Can you work these out from the model? Positions are in its coordinate system, mm. A direction names the side the tool comes from. Coordinates: 2 decimals unless noted, no trailing zeros. Order: outer loops, then holes, each group sorted by start corner. A loop starts at its lowest first (then second) coordinate and runs counter-clockwise, first axis right, second up. Notation, with made-up numbers: (-27, 52.5) - (-9, 52.5) arc R9 ccw to (-9, 69.5) - close; hole circle Ø8 at (48, -9). An arc over 180 degrees is marked (long way). Return JSON: item names as keys, results as strings. Group by question number.
1) Imagine slicing it at D-D (y = 6). Write out the boundary of the cut face in (x, z).
2) If we mould it in two halves opening along Z, with no side actions, what happens to faces 4 (the face through (0, 5, 0)), 5 (the face through (1.74, 5.26, -2.52)), 6 (the face through (1.7, -3.1, 0.1))? For each: pulls with the +Z half, pulls with the -Z half, needs draft (parallel to the pull), parting line crosses it, or undercut.
3) If I drill on line 1 along Y through (x, z) = (1.5, 0); line 2 along Z through (x, y) = (1.4, 4.25); line 3 along X through (y, z) = (6, -0.5), over which ranges is the centre line in solid material (lowest first)?
4) Imagine slicing it at B-B (x = 0.5). Write out the boundary of the cut face in (y, z), and give its area (3 significant figures).
5) Imagine slicing it at A-A (x = 1.15). Write out the boundary of the cut face in (y, z).
6) For pin 1 Ø5 at (y, z) = (4.5, 1) entering from +X; pin 2 Ø3 at (y, z) = (-1.5, -3) entering from -X; pin 3 Ø2 at (x, z) = (1.5, 3) entering from -Y; pin 4 Ø0.8 at (x, y) = (1, -5) entering from -Z, each with a flat end and sliding along its axis, tell me the tip position at first contact or that it passes through.
7) Which directions (+Z, -Z, +X, -X, +Y, -Y) give clear straight access to the entire face, cutting with the end or side of a thin tool? Please do faces 1 (the face through (2, -5, 0)), 2 (the face through (1, -5, 1)), 3 (the face through (2, 5, 0)).
8) Imagine slicing it at C-C (z = -3.5). Write out the boundary of the cut face in (x, y), and give its area (3 significant figures).
```python
from build123d import *

# Parameters (mm, degrees)
CHAMFER_1_SIZE           = 0.5
CHAMFER_1_SIZE2          = 0.288675135
CUT_EXTRUDE_1_DEPTH      = 2.5
M3X0_51_AT_2_COUNT       = 2
M3X0_51_AT_2_PITCH       = 10
M3X0_51_AT_3_COUNT       = 2
M3X0_51_AT_3_PITCH       = 14.142135624
M3X0_51_AT_4_COUNT       = 2
M3X0_51_AT_4_PITCH       = 10
SKETCH_7_W               = 2
SKETCH_7_H               = 3
SKETCH_8_OUTSIDE_W       = 20.06
SKETCH_8_OUTSIDE_H       = 20.06
CUT_EXTRUDE_2_DEPTH      = 2.2
SKETCH_9_W               = 1.5
SKETCH_9_H               = 6
CUT_EXTRUDE_3_DEPTH      = 10
CUT_EXTRUDE_4_DEPTH      = 8
CUT_EXTRUDE_4_DEPTH_BACK = 8


with BuildPart() as part:
    # Эскиз1 → Повернуть1 (revolve)
    with BuildSketch(Plane.XY):
        Polygon((0, 1.5), (0, 10), (2, 10), (2, 4.5), (4.5, 4.5), (4.5, 2.5), (2, 2.5), (2, 3.1), (1, 3.1), (1, 1.5), align=None)
    revolve(axis=Axis((0, 0, 0), (1, 0, 0)))

    # Фаска1
    chamfer_1_edges = [part.edges().sort_by_distance(p)[0] for p in [
        (4.5, -2.5, 0),
    ]]
    chamfer_1_side = [part.faces().sort_by_distance(p)[0] for p in [
        (4.5, -4.372720779, 0),
    ]]
    chamfer(chamfer_1_edges, length=CHAMFER_1_SIZE, length2=CHAMFER_1_SIZE2, reference=chamfer_1_side[0])

    # Эскиз3 → Вырез-Вытянуть1 (cut)
    with BuildSketch(Plane(origin=(4.5, 0, 0), x_dir=(0, 0, -1), z_dir=(1, 0, 0))):
        Polygon((0, 2.45), (0.350933054, 2.777921164), (0.609290224, 2.373028745), (1.030748748, 2.60337416), (1.180296502, 2.146951366), (1.645798706, 2.265247584), (1.67714041, 1.785973137), (2.15743708, 1.784787171), (2.068603417, 1.312775648), (2.533515747, 1.192182016), (2.330088465, 0.757091636), (2.750404302, 0.524667681), (2.445165485, 0.153836773), (2.79447484, -0.175813455), (2.406603764, -0.459084221), (2.662958246, -0.865247584), (2.216826279, -1.043159264), (2.364118191, -1.500315026), (1.887757445, -1.561688775), (1.916731897, -2.041112157), (1.440073868, -1.982091636), (1.348910287, -2.453658704), (0.901905154, -2.27795239), (0.696331684, -2.712032851), (0.307066422, -2.430681018), (0, -2.8), (-0.307066422, -2.430681018), (-0.696331684, -2.712032851), (-0.901905154, -2.27795239), (-1.348910287, -2.453658704), (-1.440073868, -1.982091636), (-1.916731897, -2.041112157), (-1.887757445, -1.561688775), (-2.364118191, -1.500315026), (-2.216826279, -1.043159264), (-2.662958246, -0.865247584), (-2.406603764, -0.459084221), (-2.79447484, -0.175813455), (-2.445165485, 0.153836773), (-2.750404302, 0.524667681), (-2.330088465, 0.757091636), (-2.533515747, 1.192182016), (-2.068603417, 1.312775648), (-2.15743708, 1.784787171), (-1.67714041, 1.785973137), (-1.645798706, 2.265247584), (-1.180296502, 2.146951366), (-1.030748748, 2.60337416), (-0.609290224, 2.373028745), (-0.350933054, 2.777921164), align=None)
    extrude(amount=-CUT_EXTRUDE_1_DEPTH, mode=Mode.SUBTRACT)

    # Эскиз6 → Отверстие обработанное метчиком M3x0.51 (revolve, cut)
    with BuildSketch(Plane(origin=(0, 5, -5), x_dir=(0, 0, 1), z_dir=(0, 1, 0))):
        Polygon((0, 0), (0, 2), (1.6, 2), (1.25, 1.754927362), (1.25, 0.245072638), (1.6, 0), align=None)
    m3x0_51 = revolve(axis=Axis((-6.35, 5, -5), (1, 0, 0)), mode=Mode.SUBTRACT)

    # Отверстие обработанное метчиком M3x0.51 at 2: Отверстие обработанное метчиком M3x0.51 ×2
    with Locations(*[(0, 0, i * M3X0_51_AT_2_PITCH) for i in range(1, M3X0_51_AT_2_COUNT)]):
        add(m3x0_51, mode=Mode.SUBTRACT)

    # Отверстие обработанное метчиком M3x0.51 at 3: Отверстие обработанное метчиком M3x0.51 ×2
    with Locations(*[Vector(0, -0.707106781, 0.707106781) * (i * M3X0_51_AT_3_PITCH) for i in range(1, M3X0_51_AT_3_COUNT)]):
        add(m3x0_51, mode=Mode.SUBTRACT)

    # Отверстие обработанное метчиком M3x0.51 at 4: Отверстие обработанное метчиком M3x0.51 ×2
    with Locations(*[(0, -i * M3X0_51_AT_4_PITCH, 0) for i in range(1, M3X0_51_AT_4_COUNT)]):
        add(m3x0_51, mode=Mode.SUBTRACT)

    # Эскиз7 → Вырез-Повернуть1 (revolve, cut)
    with BuildSketch(Plane.XY):
        with Locations((1, 8.5)):
            Rectangle(SKETCH_7_W, SKETCH_7_H)
    revolve(axis=Axis((0, 0, 0), (1, 0, 0)), mode=Mode.SUBTRACT)

    # Эскиз8 outside → Вырез-Вытянуть2 (cut)
    with BuildSketch(Plane.ZY):
        Rectangle(SKETCH_8_OUTSIDE_W, SKETCH_8_OUTSIDE_H)
        Polygon((-0.827225118, 6.950949475), (-4.5, 3.278174593), (-4.5, -3.278174593), (-0.827225118, -6.950949475), (-0.827225118, -8.301176924), (0.827225118, -8.301176924), (0.827225118, -6.950949475), (4.5, -3.278174593), (4.5, 3.278174593), (0.827225118, 6.950949475), (0.827225118, 9.049308712), (-0.827225118, 9.049308712), align=None, mode=Mode.SUBTRACT)
    extrude(amount=-CUT_EXTRUDE_2_DEPTH, mode=Mode.SUBTRACT)

    # Эскиз9 → Вырез-Вытянуть3 (cut, through all)
    with BuildSketch(Plane(origin=(0, 0, -4.5), x_dir=(-1, 0, 0), z_dir=(0, 0, -1))):
        with Locations((-0.75, 0)):
            Rectangle(SKETCH_9_W, SKETCH_9_H)
    extrude(amount=-CUT_EXTRUDE_3_DEPTH, mode=Mode.SUBTRACT)

    # Эскиз10 → Вырез-Вытянуть4 (cut, two sides)
    with BuildSketch(Plane(origin=(0, 0, 0), x_dir=(1, 0, 0), z_dir=(0, 1, 0))) as cut_extrude_4_sk:
        Polygon((0, -1), (0, 1), (1.5, 1), (1.5, 5.512863142), (-0.606676523, 5.512863142), (-0.606676523, -5.078399816), (1.5, -5.078399816), (1.5, -1), align=None)
    extrude(amount=CUT_EXTRUDE_4_DEPTH, mode=Mode.SUBTRACT)
    extrude(cut_extrude_4_sk.sketch, amount=-CUT_EXTRUDE_4_DEPTH_BACK, mode=Mode.SUBTRACT)


solid = part.part
```
Calculated:
{
 "1": {"outline": "(0, -1) - (1.5, -1) - (1.5, -1.78) - (2, -1.78) - (2, 1.78) - (1.5, 1.78) - (1.5, 1) - (0, 1) - close"},
 "2": {"face 4": "needs draft", "face 5": "pulls with the -Z half", "face 6": "undercut"},
 "3": {"line 1": "-7 to -3.1, 3.1 to 7", "line 2": "-1 to 1", "line 3": "0 to 2"},
 "4": {"outline": "(-6.95, -0.83) - (-6.78, -1) - (-3, -1) - (-3, 1) - (-6.78, 1) - (-6.95, 0.83) arc R7 ccw to start; (3, -1) - (6.78, -1) - (6.95, -0.83) arc R7 ccw to (6.95, 0.83) - (6.78, 1) - (3, 1) - close", "area": "15.9 mm2"},
 "5": {"outline": "(-6.95, -0.83) - (-6.78, -1) - (-3, -1) - (-3, -0.78) arc R3.1 cw to (-3, 0.78) - (-3, 1) - (-6.78, 1) - (-6.95, 0.83) arc R7 ccw to start; (3, -1) - (6.78, -1) - (6.95, -0.83) arc R7 ccw to (6.95, 0.83) - (6.78, 1) - (3, 1) - (3, 0.78) arc R3.1 cw to (3, -0.78) - close"},
 "6": {"pin 1": "x = 4.5", "pin 2": "x = 1.5", "pin 3": "y = -5.78", "pin 4": "z = -1"},
 "7": {"face 1": "+X, -Y", "face 2": "+Z, -X, +Y, -Y", "face 3": "+X, +Y"},
 "8": {"outline": "(1.5, -4.28) - (2, -4.28) - (2, -2.83) - (4.5, -2.83) - (4.5, 2.83) - (2, 2.83) - (2, 4.28) - (1.5, 4.28) - close", "area": "18.4 mm2"}
}
